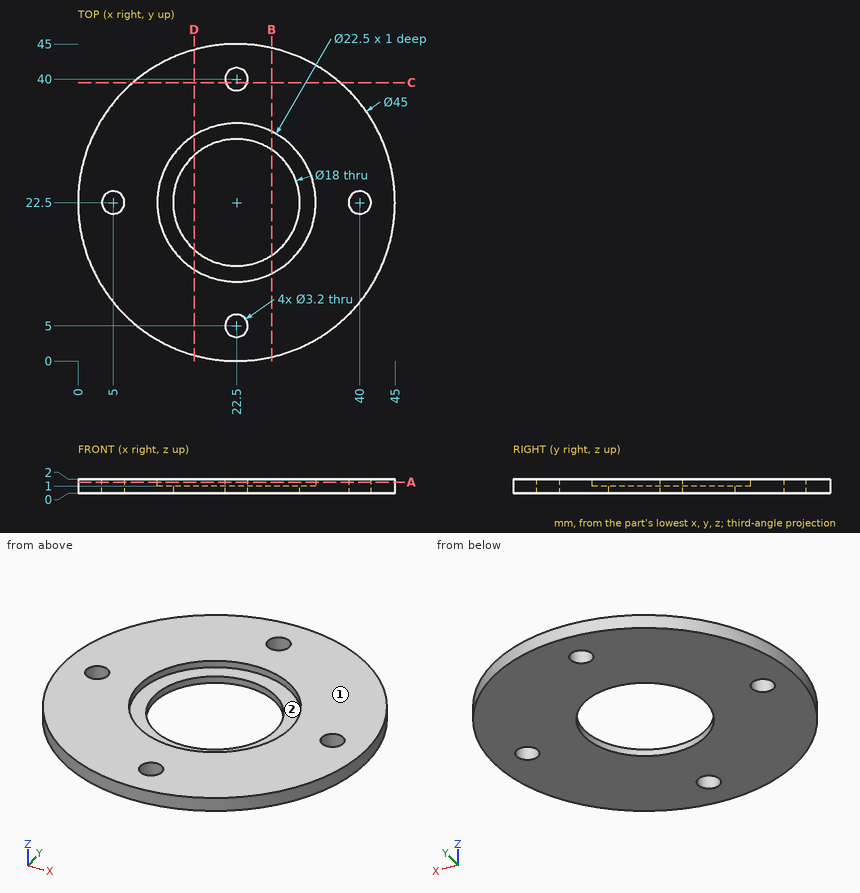
For this review, use the dimensioned drawing (mm, ordinates from the lowest corner) and the shaded views. A direction names the side the tool comes from. Give positions to 0.01 mm unless a question says otherwise; leave off trailing zeros. Order: outer loops, then holes, each group sorted by start corner. A loop starts at its lowest first (then second) coordinate and runs counter-clockwise, first axis right, second up.
1. Add section D-D, the plane x = 16.5. State the section outline as (y, z) points, then the cut area to 3 significant figures.
Solution:
outline: (0.81, 0) - (15.79, 0) - (15.79, 1) - (12.98, 1) - (12.98, 2) - (0.81, 2) - close; (29.21, 0) - (44.19, 0) - (44.19, 2) - (32.02, 2) - (32.02, 1) - (29.21, 1) - close
area: 54.3 mm2
2. Tool access review of the marked faces 1 and 2: name each direction out of +Z, -Z, +X, -X, +Y, -Y from which nothing blocks a thin tool from reaching the whole face with its end or side.
Solution:
face 1: +Z, +X, -X, +Y, -Y
face 2: +Z
3. Add section B-B, the plane x = 27.5. State the section outline as (y, z) points, then the cut area to 3 significant figures.
Solution:
outline: (0.56, 0) - (15.02, 0) - (15.02, 1) - (12.42, 1) - (12.42, 2) - (0.56, 2) - close; (29.98, 0) - (44.44, 0) - (44.44, 2) - (32.58, 2) - (32.58, 1) - (29.98, 1) - close
area: 52.6 mm2
4. For pin 1 Ø20 at (x, y) = (22.5, 22.5) entering from +Z; pin 2 Ø14.5 at (x, y) = (22.5, 22.5) entering from -Z, all flat-tipped, find the tip position at first contact; note any pin that passes through.
Solution:
pin 1: stops at z = 1
pin 2: passes through
5. Add section C-C, the plane y = 39.5. State the section outline as (x, z) points, then the cut area to 3 significant figures.
Solution:
outline: (7.76, 0) - (20.98, 0) - (20.98, 2) - (7.76, 2) - close; (24.02, 0) - (37.24, 0) - (37.24, 2) - (24.02, 2) - close
area: 52.9 mm2
6. Add section A-A, the plane z = 1.55. State the section outline as (x, y) points.
Solution:
outline: circle Ø45 at (22.5, 22.5); hole circle Ø3.2 at (5, 22.5); hole circle Ø22.5 at (22.5, 22.5); hole circle Ø3.2 at (22.5, 5); hole circle Ø3.2 at (22.5, 40); hole circle Ø3.2 at (40, 22.5)
7. To check wall thickness, follow L1, parallel to X at y = 22, z = 1.95; L2, parallel to X at y = 18, z = 1.7; L3, parallel to X at y = 5, z = 1.55. State the ranges of each line that lie inside material, in increasing order.
Solution:
L1: x = 0.01 to 3.48, 6.52 to 11.26, 33.74 to 38.48, 41.52 to 44.99
L2: x = 0.45 to 12.19, 32.81 to 44.55
L3: x = 8.36 to 20.9, 24.1 to 36.64
